Geometry check sheet. Reference: the model listing, model coordinates, mm. Face numbers are marked on the shaded views. A direction names the side the tool comes from. Give positions to 0.01 mm unless a question says otherwise; leave off trailing zeros. Loops run counter-clockwise (first coordinate to the right, second up) from the corner with the lowest first, then second, coordinate; pieces in that order, holes last. Notation, with made-up numbers: (-33.75, 12.25) -> (8.25, 12.25) arc R25 cw to (8.25, 43.25) -> close; hole circle Ø11 at (-11, 63.5). An arc over 180 degrees is marked (long way). Answer as a JSON object with one key per item and string values.
from build123d import *

# Parameters (mm, degrees)
SKETCH_1_W          = 12
SKETCH_1_H          = 25
SKETCH_1_R          = 1.75
EXTRUDE_1_DEPTH     = 20
CUT_EXTRUDE_1_DEPTH = 26
SKETCH_3_R          = 3
CUT_EXTRUDE_2_DEPTH = 10
SKETCH_4_R          = 3.75
CUT_EXTRUDE_3_DEPTH = 3


with BuildPart() as part:
    # Эскиз1 → Бобышка-Вытянуть1 (new body)
    with BuildSketch(Plane(origin=(0, 0, 0), x_dir=(1, 0, 0), z_dir=(0, 1, 0))):
        with Locations((6, 12.5)):
            Rectangle(SKETCH_1_W, SKETCH_1_H)
        with Locations((7, 6)):
            Circle(SKETCH_1_R, mode=Mode.SUBTRACT)
        with Locations((7, 16)):
            Circle(SKETCH_1_R, mode=Mode.SUBTRACT)
    extrude(amount=EXTRUDE_1_DEPTH)

    # Эскиз2 → Вырез-Вытянуть1 (cut, through all)
    with BuildSketch(Plane.XY):
        Polygon((-54.72135955, 14), (0, 14), (3, 14), (3, 15.6), (2, 15.6), (2, 20), (2, 74.72135955), (-77.977073961, 149.429969527), (-134.698433511, 88.708609977), align=None)
    extrude(amount=-CUT_EXTRUDE_1_DEPTH, mode=Mode.SUBTRACT)

    # Эскиз3 → Вырез-Вытянуть2 (cut)
    with BuildSketch(Plane(origin=(0, 20, 0), x_dir=(1, 0, 0), z_dir=(0, 1, 0))):
        with Locations((7, 16)):
            Circle(SKETCH_3_R)
        with Locations((7, 6)):
            Circle(SKETCH_3_R)
    extrude(amount=-CUT_EXTRUDE_2_DEPTH, mode=Mode.SUBTRACT)

    # Эскиз4 → Вырез-Вытянуть3 (cut)
    with BuildSketch(Plane.XZ):
        with Locations((7, -16)):
            Circle(SKETCH_4_R)
        with Locations((7, -6)):
            Circle(SKETCH_4_R)
    extrude(amount=-CUT_EXTRUDE_3_DEPTH, mode=Mode.SUBTRACT)


solid = part.part
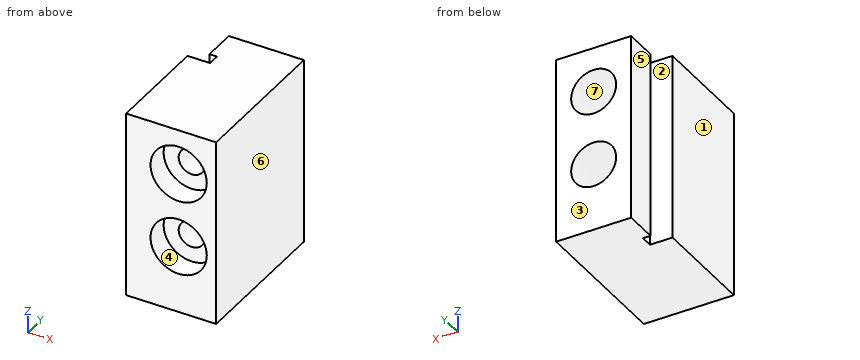
1) Depth check by flat-ended pin: P1, Ø1.5, axis at x = 1, z = -18.5, coming from the +Y side; P2, Ø3.5, axis at y = 17, z = -10.5, coming from the -X side; P3, Ø4, axis at x = 7.5, z = -16.5, coming from the -Y side; P4, Ø3, axis at x = 7, z = -6, coming from the +Y side. Enter the tip coordinate at first touch or a pass-through.
Geometry check:
{"P1": "stops at y = 14", "P2": "stops at x = 2", "P3": "stops at y = 3", "P4": "passes through"}
2) Tool access check on the marked faces 4, 5, 6 and 7. Record the directions out of +Z, -Z, +X, -X, +Y, -Y that give a thin tool (end or side, any length) a straight path to the whole face; none if there is none.
Geometry check:
{"face 4": "-Y", "face 5": "+Z, -Z, -X, +Y", "face 6": "+Z, -Z, +X, +Y, -Y", "face 7": "+Y"}
3) Section check B-B on z = -6. Record the cut outline in (x, y), plus the area to 3 significant figures.
Geometry check:
{"outline": "(0, 0) -> (3.25, 0) -> (3.25, 3) -> (5.25, 3) -> (5.25, 10) -> (4, 10) -> (4, 20) -> (2, 20) -> (2, 15.6) -> (3, 15.6) -> (3, 14) -> (0, 14) -> close; (8.75, 3) -> (10.75, 3) -> (10.75, 0) -> (12, 0) -> (12, 20) -> (10, 20) -> (10, 10) -> (8.75, 10) -> close", "area": "119 mm2"}
4) Draft check along Y on the marked faces 1, 2 and 3. Enter one of: pulls with the +Y half, pulls with the -Y half, needs draft (parallel to the pull), parting line crosses it, or undercut.
Geometry check:
{"face 1": "needs draft", "face 2": "undercut", "face 3": "pulls with the +Y half"}
5) Section check C-C on y = 17.75. Record the cut outline in (x, z).
Geometry check:
{"outline": "(2, -25) -> (12, -25) -> (12, 0) -> (2, 0) -> close; hole circle Ø6 at (7, -16); hole circle Ø6 at (7, -6)"}
6) Material ranges on line 1 along Z through (x, y) = (7, 1.7); line 2 along Z through (x, y) = (7, 17); line 3 along X through (y, z) = (12.75, -6), recorded low to high. Write a range as from..to.
Geometry check:
{"line 1": "z = -25..-19.75, -12.25..-9.75, -2.25..0", "line 2": "z = -25..-19, -13..-9, -3..0", "line 3": "x = 0..4, 10..12"}
7) Section check D-D on z = -23.25. Record the cut outline in (x, y).
Geometry check:
{"outline": "(0, 0) -> (12, 0) -> (12, 20) -> (2, 20) -> (2, 15.6) -> (3, 15.6) -> (3, 14) -> (0, 14) -> close"}
8) Section check A-A on x = 7. Record the cut outline in (y, z).
Geometry check:
{"outline": "(0, -25) -> (20, -25) -> (20, -19) -> (10, -19) -> (10, -17.75) -> (3, -17.75) -> (3, -19.75) -> (0, -19.75) -> close; (0, -12.25) -> (3, -12.25) -> (3, -14.25) -> (10, -14.25) -> (10, -13) -> (20, -13) -> (20, -9) -> (10, -9) -> (10, -7.75) -> (3, -7.75) -> (3, -9.75) -> (0, -9.75) -> close; (0, -2.25) -> (3, -2.25) -> (3, -4.25) -> (10, -4.25) -> (10, -3) -> (20, -3) -> (20, 0) -> (0, 0) -> close"}
